Build history of the part. All positions in model axes, mm. A direction names the side the tool comes from. Round coordinates to 2 decimals unless told otherwise and drop trailing zeros. Write each loop counter-clockwise with the first axis right and the second up, starting at its lowest first coordinate (ties: lowest second). Pieces come first, ordered by that corner, then holes. Notation, with made-up numbers: M 9.25,40 L 63.25,40 A19 ccw 63.25,70 Z; hole C 73,47.5 d8. An arc over 180 degrees is marked long. One line per item, written item: value. Start each with the question number.
```python
from build123d import *

# Parameters (mm, degrees)
SKETCH1_W      = 35.9
SKETCH1_H      = 17.8
EXTRUDE1_DEPTH = 1.7
SKETCH2_W      = 9
SKETCH2_H      = 7.7
EXTRUDE2_DEPTH = 3.75
SKETCH3_W      = 35.9
SKETCH3_H      = 2.6
EXTRUDE3_DEPTH = 8.4


with BuildPart() as part:
    # Sketch1 → Extrude1 (new body)
    with BuildSketch(Plane(origin=(0, 0, 0), x_dir=(1, 0, 0), z_dir=(0, 1, 0))):
        with Locations((-38.756784273, 20.763622827)):
            Rectangle(SKETCH1_W, SKETCH1_H)
    extrude(amount=EXTRUDE1_DEPTH)

    # Sketch2 → Extrude2 (add)
    with BuildSketch(Plane(origin=(0, 1.7, 0), x_dir=(1, 0, 0), z_dir=(0, 1, 0))):
        with Locations((-53.206784273, 20.763622827)):
            Rectangle(SKETCH2_W, SKETCH2_H)
    extrude(amount=EXTRUDE2_DEPTH)

    # Sketch3 → Extrude3 (add)
    with BuildSketch(Plane.XZ):
        with Locations((-38.756784273, -13.163622827)):
            Rectangle(SKETCH3_W, SKETCH3_H)
        with Locations((-38.756784273, -28.363622827)):
            Rectangle(SKETCH3_W, SKETCH3_H)
    extrude(amount=EXTRUDE3_DEPTH)


solid = part.part
```
Item 1: Drill centre lines: line 1 (Z direction, x = -28, y = -3.5); line 2 (Y direction, x = -24, z = -15.75); line 3 (Z direction, x = -52.5, y = 4.75). Where is each one in solid material? Low to high.
Item 2: Drop flat-ended pins along their axis: pin 1 (4 mm diameter, centred on x = -33.5, z = -13.5, fed in from +Y); pin 2 (1.1 mm diameter, centred on x = -53, y = 4, fed in from +Z); pin 3 (8 mm diameter, centred on y = -3, z = -24, fed in from -X). Give the stop position or say it passes through.
Item 3: Cut at B-B, the plane x = -53.5. Write the cut outline in (y, z), plus the area to 3 significant figures.
Item 4: Cut at A-A, the plane y = -6. Write the cut outline in (x, z), plus the area to 3 significant figures.
Item 5: Cut at C-C, the plane z = -19.25. Write the cut outline in (x, y).
Item 6: Which spindle directions (+Z, -Z, +X, -X, +Y, -Y) get a long thin tool onto all of the face, cutting with end or side? Do faces 1 (the flat face through (-53, 4, -24.614)), 2 (the flat face through (-39, -4, -14.464)), 3 (the flat face through (-48.707, 4, -21)). Say none if no direction does.
Item 7: Cut at D-D, the plane x = -25.5. Write the cut outline in (y, z).
Computed values:
1. line 1: z = -29.66 to -27.06, -14.46 to -11.86
1. line 2: y = 0 to 1.7
1. line 3: z = -24.61 to -16.91
2. pin 1: stops at y = 1.7
2. pin 2: stops at z = -16.91
2. pin 3: stops at x = -56.71
3. outline: M -8.4,-29.66 L 1.7,-29.66 L 1.7,-24.61 L 5.45,-24.61 L 5.45,-16.91 L 1.7,-16.91 L 1.7,-11.86 L -8.4,-11.86 L -8.4,-14.46 L 0,-14.46 L 0,-27.06 L -8.4,-27.06 Z
3. area: 103 mm2
4. outline: M -56.71,-29.66 L -20.81,-29.66 L -20.81,-27.06 L -56.71,-27.06 Z; M -56.71,-14.46 L -20.81,-14.46 L -20.81,-11.86 L -56.71,-11.86 Z
4. area: 187 mm2
5. outline: M -57.71,1.7 L -56.71,1.7 L -56.71,0 L -20.81,0 L -20.81,1.7 L -48.71,1.7 L -48.71,5.45 L -57.71,5.45 Z
6. face 1: -Z, +X, -X, +Y
6. face 2: +X, -X, -Y
6. face 3: +Z, -Z, +X, +Y
7. outline: M -8.4,-29.66 L 1.7,-29.66 L 1.7,-11.86 L -8.4,-11.86 L -8.4,-14.46 L 0,-14.46 L 0,-27.06 L -8.4,-27.06 Z
